Build history of the part. All positions in model axes, mm. Give positions to 0.01 mm unless a question says otherwise; leave off trailing zeros. Order: outer loops, then holes, each group sorted by start corner. A loop starts at its lowest first (then second) coordinate and runs counter-clockwise, first axis right, second up. Notation, with made-up numbers: (-29.5, 77.5) -> (-20.5, 77.5) arc R13 cw to (-20.5, 84.5) -> close; hole circle Ø8 at (51, 2). An arc over 180 degrees is marked (long way). One line per item, written item: value. Start each with the question number.
(1) Saw through at C-C on x = -102. Give the cut face in (y, z), plus the area to 3 significant figures.
(2) Probe line 1 (X direction, y = 122.5, z = 4.25); line 2 (X direction, y = 67, z = 1.65); line 3 (X direction, y = 11, z = 2.35). List the from-to ranges inside material, lowest first.
(3) Pin check, flat tips, straight feed: pin 1 (3 mm diameter, centred on y = 39.5, z = 5, fed in from -X); pin 2 (1.8 mm diameter, centred on x = -4.5, z = 3.5, fed in from +Y); pin 3 (1.8 mm diameter, centred on x = -143.5, z = 3, fed in from +Y). Stop position of each tip, or through.
(4) Saw through at D-D on y = 26.5. Give the cut face in (x, z).
(5) Saw through at A-A on y = 60. Give the cut face in (x, z), plus the area to 3 significant figures.
(6) Saw through at B-B on z = 2.75. Count the separate pieces of the cut face and the enclosed holes in it, plus the area to 3 significant figures.
```python
from build123d import *

# Parameters (mm, degrees)
ESQUISSE1_W                  = 175
ESQUISSE1_H                  = 180
BOSS_EXTRU_1_DEPTH           = 6
ESQUISSE2_W                  = 6
ESQUISSE2_H                  = 26
ESQUISSE2_W_2                = 45
ESQUISSE2_H_2                = 6
ESQUISSE2_H_3                = 90
ENL_V_MAT_ENCOCHE_DEPTH      = 252.119493469
ESQUISSE3_W                  = 6
ESQUISSE3_H                  = 20
ENL_V_MAT_ENCOCHE_TAGE_DEPTH = 6


with BuildPart() as part:
    # Esquisse1 → Boss.-Extru.1 (new body)
    with BuildSketch(Plane.XY):
        with Locations((-87.5, 90)):
            Rectangle(ESQUISSE1_W, ESQUISSE1_H)
    extrude(amount=BOSS_EXTRU_1_DEPTH)

    # Esquisse2 → Enl_v. mat encoche (cut, through all)
    with BuildSketch(Plane.XY.offset(6)):
        Polygon((0, 180), (-6, 180), (-45, 180), (-45, 174), (-6, 174), (-6, 143), (0, 143), align=None)
        with Locations((-3, 90)):
            Rectangle(ESQUISSE2_W, ESQUISSE2_H)
        Polygon((0, 0), (-6, 0), (-45, 0), (-45, 6), (-6, 6), (-6, 37), (0, 37), align=None)
        Polygon((-175, 0), (-130, 0), (-130, 6), (-169, 6), (-169, 20), (-175, 20), (-175, 6), align=None)
        with Locations((-87.5, 3)):
            Rectangle(ESQUISSE2_W_2, ESQUISSE2_H_2)
        Polygon((-175, 174), (-175, 150), (-169, 150), (-169, 174), (-130, 174), (-130, 180), (-175, 180), align=None)
        with Locations((-172, 75)):
            Rectangle(ESQUISSE2_W, ESQUISSE2_H_3)
        with Locations((-87.5, 177)):
            Rectangle(ESQUISSE2_W_2, ESQUISSE2_H_2)
    extrude(amount=-ENL_V_MAT_ENCOCHE_DEPTH, mode=Mode.SUBTRACT)

    # Esquisse3 → Enlèv. mat encoche étage (cut)
    with BuildSketch(Plane.XY.offset(6)):
        with Locations((-52, 120)):
            Rectangle(ESQUISSE3_W, ESQUISSE3_H)
        with Locations((-52, 60)):
            Rectangle(ESQUISSE3_W, ESQUISSE3_H)
    extrude(amount=-ENL_V_MAT_ENCOCHE_TAGE_DEPTH, mode=Mode.SUBTRACT)


solid = part.part
```
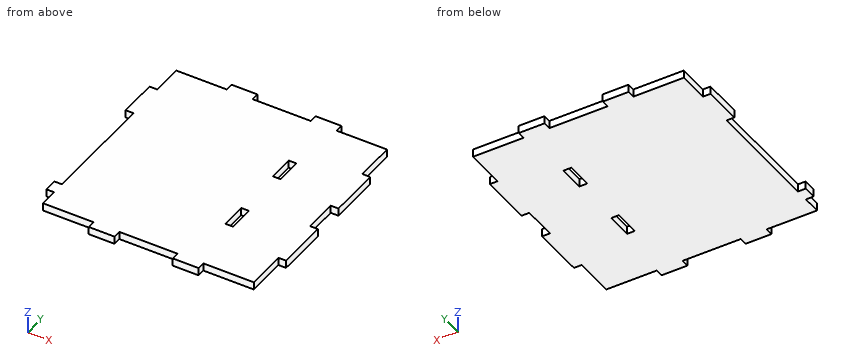
Results below:
1. outline: (6, 0) -> (174, 0) -> (174, 6) -> (6, 6) -> close
1. area: 1,010 mm²
2. line 1: x = -175 to -55, -49 to 0
2. line 2: x = -169 to -55, -49 to 0
2. line 3: x = -169 to -6
3. pin 1: stops at x = -169
3. pin 2: stops at y = 143
3. pin 3: stops at y = 174
4. outline: (-175, 0) -> (-6, 0) -> (-6, 6) -> (-175, 6) -> close
5. outline: (-169, 0) -> (-55, 0) -> (-55, 6) -> (-169, 6) -> close; (-49, 0) -> (0, 0) -> (0, 6) -> (-49, 6) -> close
5. area: 978 mm²
6. separate pieces: 1
6. enclosed holes: 2
6. area: 28,300 mm²
